Source: CAD feature listing. Evaluate the final solid. Frame: model axes, mm. A direction names the side the tool comes from. Round coordinates to 2 decimals unless told otherwise and drop trailing zeros. Write each loop counter-clockwise with the first axis right and the second up, starting at its lowest first coordinate (ties: lowest second). Pieces come first, ordered by that corner, then holes. Notation, with made-up numbers: M 46.25,87.5 L 89.25,87.5 A4 cw 89.25,92.5 Z; hole C 58.5,6.5 d3. An arc over 180 degrees is marked long. Answer in a Markdown table with one row per item.
from build123d import *

# Parameters (mm, degrees)
EXTRUDE_2_DEPTH     = 2
SKETCH_3_R          = 1.5
CUT_EXTRUDE_1_DEPTH = 95.361008897
EXTRUDE_3_DEPTH     = 1
DRAFT_4_ANGLE       = 43


with BuildPart() as part:
    # 草图1 → 凸台-拉伸2 (new body)
    with BuildSketch(Plane.XY):
        Polygon((0, 0), (0, 50), (20, 50), (20, 40), (60, 40), (60, 50), (80, 50), (80, 0), (60, 0), (60, 10), (20, 10), (20, 0), align=None)
    extrude(amount=EXTRUDE_2_DEPTH)

    # 草图3 → 切除-拉伸1 (cut, through all)
    with BuildSketch(Plane.XY.offset(2)):
        with Locations((10, 45)):
            Circle(SKETCH_3_R)
        with Locations((10, 5)):
            Circle(SKETCH_3_R)
        with Locations((70, 45)):
            Circle(SKETCH_3_R)
        with Locations((70, 5)):
            Circle(SKETCH_3_R)
    extrude(amount=-CUT_EXTRUDE_1_DEPTH, mode=Mode.SUBTRACT)

    # 草图5 → 凸台-拉伸3 (add)
    with BuildSketch(Plane.XY.offset(2)):
        with BuildLine():
            Line((0, 50), (6, 50))
            Line((6, 50), (6, 45))
            ThreePointArc((6, 45), (10, 41), (14, 45))
            Line((14, 45), (14, 50))
            Line((14, 50), (20, 50))
            Line((20, 50), (20, 40))
            Line((20, 40), (60, 40))
            Line((60, 40), (60, 50))
            Line((60, 50), (66, 50))
            Line((66, 50), (66, 45))
            ThreePointArc((66, 45), (70, 41), (74, 45))
            Line((74, 45), (74, 50))
            Line((74, 50), (80, 50))
            Line((80, 50), (80, 0))
            Line((80, 0), (74, 0))
            Line((74, 0), (74, 5))
            ThreePointArc((74, 5), (70, 9), (66, 5))
            Line((66, 5), (66, 0))
            Line((66, 0), (60, 0))
            Line((60, 0), (60, 10))
            Line((60, 10), (20, 10))
            Line((20, 10), (20, 0))
            Line((20, 0), (14, 0))
            Line((14, 0), (14, 5))
            ThreePointArc((14, 5), (10, 9), (6, 5))
            Line((6, 5), (6, 0))
            Line((6, 0), (0, 0))
            Line((0, 0), (0, 50))
        make_face()
    extrude(amount=EXTRUDE_3_DEPTH)

    # 拔模4
    draft_4_faces = [part.faces().sort_by_distance(p)[0] for p in [
        (40, 25, 3),
    ]]
    draft(draft_4_faces, Plane(origin=(20, 0, 2), x_dir=(-1, 0, 0), z_dir=(0, -1, 0)), DRAFT_4_ANGLE)


solid = part.part
Q1. Section A-A (x = 10). Return loops of the section in (y, z).
Solutions:
| item | result |
|---|---|
| outline | M 0,0 L 3.5,0 L 3.5,2 L 0,2 Z; M 6.5,0 L 43.5,0 L 43.5,2 L 41,2 L 41,41.23 L 9,11.39 L 9,2 L 6.5,2 Z; M 46.5,0 L 50,0 L 50,2 L 46.5,2 Z |
Q2. Section B-B (z = 6). Return loops of the section in (x, y), and give its area (3 significant figures).
Solutions:
| item | result |
|---|---|
| outline | M 0,3.22 L 6,3.22 L 6,5 A4 cw 14,5 L 14,3.22 L 20,3.22 L 20,10 L 60,10 L 60,3.22 L 66,3.22 L 66,5 A4 cw 74,5 L 74,3.22 L 80,3.22 L 80,50 L 74,50 L 74,45 A4 cw 66,45 L 66,50 L 60,50 L 60,40 L 20,40 L 20,50 L 14,50 L 14,45 A4 cw 6,45 L 6,50 L 0,50 Z |
| area | 2,860 mm2 |
Q3. Pull-direction query (X, two-part tool) for faces 6 (the flat face through (74.3, 50, 24.5)), 7 (the cylindrical face through (10, 9, 6)), 8 (the flat face through (80, 31, 19)), 9 (the cylindrical face through (10, 41, 23)); classes: pulls with the +X half, pulls with the -X half, needs draft (parallel to the pull), parting line crosses it, or undercut.
Solutions:
| item | result |
|---|---|
| face 6 | needs draft |
| face 7 | undercut |
| face 8 | pulls with the +X half |
| face 9 | undercut |
Q4. Section D-D (y = 29.5). Return loops of the section in (x, z), and give its area (3 significant figures).
Solutions:
| item | result |
|---|---|
| outline | M 0,0 L 80,0 L 80,30.51 L 0,30.51 Z |
| area | 2,440 mm2 |
Q5. Contact query for flat-ended pins moving along their axis: pin 1 Ø1.5 at (x, z) = (24.5, 19) entering from -Y; pin 2 Ø8 at (x, y) = (66.5, 42.5) entering from +Z; pin 3 Ø1.5 at (x, z) = (39.5, 38.5) entering from +Y; pin 4 Ø2.5 at (x, y) = (10, 45) entering from +Z. Output: stop coordinate, or through.
Solutions:
| item | result |
|---|---|
| pin 1 | stops at y = 16.35 |
| pin 2 | stops at z = 46.33 |
| pin 3 | stops at y = 40 |
| pin 4 | passes through |
Q6. Access query for faces 1 (the flat face through (40, 40, 20)), 2 (the cylindrical face through (9.675, 43.536, 1.014)), 3 (the flat face through (41, 25, 0)), 4 (the flat face through (70, 47, 2)), 5 (the cylindrical face through (70, 9, 6)). Directions: +Z, -Z, +X, -X, +Y, -Y. A direction counts if a zero-diameter tool reaches every point of the face in a straight line with its end or side. Return the directions, or none.
Solutions:
| item | result |
|---|---|
| face 1 | +Z, -Z, +Y |
| face 2 | +Z, -Z |
| face 3 | -Z, +X, -X, +Y, -Y |
| face 4 | +Z, +Y |
| face 5 | +Z, -Y |
Q7. Material intervals for probe 1 along Y at (x, z) = (10, 0.9); probe 2 along X at (y, z) = (42, 21.5); probe 3 along Y at (x, z) = (10, 3.5), sorted ascending.
Solutions:
| item | result |
|---|---|
| probe 1 | y = 0 to 3.5, 6.5 to 43.5, 46.5 to 50 |
| probe 2 | x = 0 to 7.35, 12.65 to 20, 60 to 67.35, 72.65 to 80 |
| probe 3 | y = 9 to 41 |
Q8. Section C-C (x = 51). Return loops of the section in (y, z).
Solutions:
| item | result |
|---|---|
| outline | M 10,0 L 40,0 L 40,40.3 L 10,12.33 Z |
